Here's how the part is built. I have some questions about the finished solid (model axes, mm). Face numbers are marked on the shaded views. A direction names the side the tool comes from. Round coordinates to 2 decimals unless told otherwise and drop trailing zeros. Loops run counter-clockwise (first coordinate to the right, second up) from the corner with the lowest first, then second, coordinate; pieces in that order, holes last. Notation, with made-up numbers: M -28,64.25 L -9,64.25 A4 cw -9,68.25 Z; hole C 2.25,89 d10. An arc over 180 degrees is marked long. Answer as a JSON object with one key per item and string values.
Autodesk Fusion 360 part; units mm, degrees
sketch "Sketch1" plane through (0, 0, 0) normal (0, 0, 1) x (1, 0, 0)
  line L0 (0, 0) -> (110, 0)
  line L1 (110, 0) -> (110, 60)
  line L2 (110, 60) -> (0, 60)
  line L3 (0, 60) -> (0, 0)
  line L4 (0, 60) -> (110, 60)
  line L5 (110, 60) -> (110, 35)
  line L6 (110, 35) -> (0, 35)
  line L7 (0, 35) -> (0, 60)
  line L8 (75, 25) -> (35, 25)
  line L9 (35, 25) -> (35, 0)
  line L10 (75, 0) -> (75, 25)
  line L11 (75, 25) -> (35, -25) construction
  line L12 (35, 25) -> (75, -25) construction
  point P0 (55, 0)
  dimension "d12" = 110
  dimension "d13" = 60
  dimension "d14" = 110
  dimension "d15" = 25
  dimension "d16" = 40
  dimension "d17" = 50
extrude "Extrude1" add sketch "Sketch1" along normal blind 30 contours L0 L1 L3 L6 L8 L9 L10
extrude "Extrude2" add sketch "Sketch1" along normal blind 80 contours L1 L2 L3 L4 L5 L6 L7
fillet "Fillet1" radius 6 2 edges at (110, 47.5, 80) (0, 47.5, 80)
chamfer "Chamfer1" distance 3 angle 45 4 edges at (110, 0, 15) (75, 0, 15) (35, 0, 15) (0, 0, 15)
sketch "Sketch2" plane through (0, 35, 0) normal (0, -1, 0) x (1, 0, 0)
  arc A0 (6, 80) -> (0, 74) centre (6, 74) ccw
  line L0 (0, 74) -> (0, 30)
  line L1 (0, 30) -> (110, 30)
  line L2 (110, 30) -> (110, 74)
  arc A1 (110, 74) -> (104, 80) centre (104, 74) ccw
  line L3 (104, 80) -> (6, 80)
  line L4 (55, 80) -> (55, 30) construction
  circle A2 centre (80, 55) radius 6
  circle A3 centre (80, 55) radius 3
  circle A4 centre (30, 55) radius 6
  circle A5 centre (30, 55) radius 3
  dimension "d27" = 12
  dimension "d28" = 6
  dimension "d29" = 25
  dimension "d32" = 25
extrude "Extrude3" cut sketch "Sketch2" against normal blind 25 contours A3 | A5
extrude "Extrude4" cut sketch "Sketch2" against normal blind 5 contours A4
extrude "Extrude5" cut sketch "Sketch2" against normal blind 5 contours A2
equation "width = 60 mm"
equation "length = 110 mm"
equation "base_height = 30 mm"
equation "back_height = 80 mm"
equation "back_width = 25 mm"
equation "countersink_diameter = 12 mm"
equation "hole_diameter = 6 mm"
equation "countersink_depth = 5 mm"
equation "cut_depth = 25 mm"
equation "cut_width = 40 mm"
equation "d12 = length"
equation "d13 = width"
equation "d14 = length"
equation "d15 = back_width"
equation "d16 = cut_width"
equation "d17 = cut_depth * 2"
equation "top_radius = 6 mm"
equation "d19 = base_height"
equation "d21 = back_height"
equation "d24 = top_radius"
equation "chamfer = 3 mm"
equation "d26 = chamfer"
equation "d27 = countersink_diameter"
equation "d28 = hole_diameter"
equation "d29 = hole_distance_from_top"
equation "hole_distance_from_top = 25 mm"
equation "distance_between_holes = 50 mm"
equation "d32 = distance_between_holes / 2"
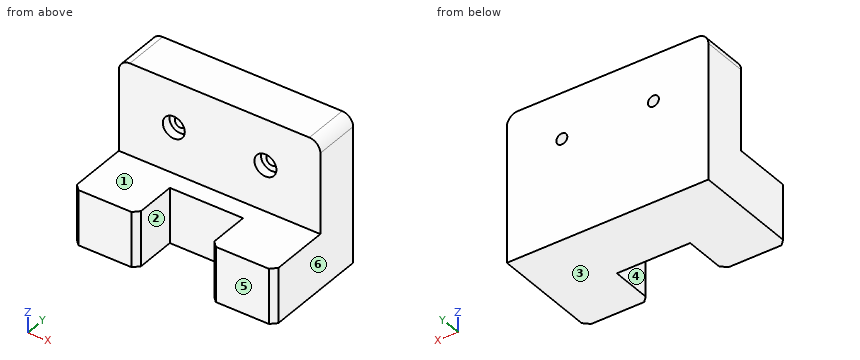
Item 1: I want a section at C-C, the plane y = 38.5. Please give me the cut outline in (x, z).
Resolved:
{"outline": "M 0,0 L 110,0 L 110,74 A6 ccw 104,80 L 6,80 A6 ccw 0,74 Z; hole C 30,55 d12; hole C 80,55 d12"}
Item 2: I want a section at A-A, the plane x = 30. Please give me the cut outline in (y, z), then the cut area to 3 significant figures.
Resolved:
{"outline": "M 0,0 L 60,0 L 60,52 L 40,52 L 40,49 L 35,49 L 35,30 L 0,30 Z; M 35,61 L 40,61 L 40,58 L 60,58 L 60,80 L 35,80 Z", "area": "2,870 mm²"}
Item 3: I'm going to push flat-ended pins straight in: pin 1 Ø3 at (x, z) = (56.5, 20) entering from -Y; pin 2 Ø3.5 at (x, z) = (31.5, 55.5) entering from -Y; pin 3 Ø4 at (x, z) = (20.5, 68) entering from -Y. Where does each tip first touch, or does it pass through?
Resolved:
{"pin 1": "y = 25", "pin 2": "y = 40", "pin 3": "y = 35"}
Item 4: On a 3-axis mill with a long thin cutter (end or side, diameter ignored), from which of +Z, -Z, +X, -X, +Y, -Y can I reach the whole of each face in a straight line? I mean the marked faces 1, 2 and 3. Say none if no direction works.
Resolved:
{"face 1": "+Z, +X, -X, -Y", "face 2": "+Z, -Z, -Y", "face 3": "-Z, +X, -X, +Y, -Y"}
Item 5: If we mould it in two halves opening along X, with no side actions, what happens to the marked faces 4, 5 and 6? For each: pulls with the +X half, pulls with the -X half, needs draft (parallel to the pull), parting line crosses it, or undercut.
Resolved:
{"face 4": "undercut", "face 5": "needs draft", "face 6": "pulls with the +X half"}
Item 6: I want a section at B-B, the plane z = 55. Please give me the cut outline in (x, y), then the cut area to 3 significant figures.
Resolved:
{"outline": "M 0,35 L 24,35 L 24,40 L 27,40 L 27,60 L 0,60 Z; M 33,40 L 36,40 L 36,35 L 74,35 L 74,40 L 77,40 L 77,60 L 33,60 Z; M 83,40 L 86,40 L 86,35 L 110,35 L 110,60 L 83,60 Z", "area": "2,390 mm²"}
Item 7: I want a section at D-D, the plane x = 72. Please give me the cut outline in (y, z), then the cut area to 3 significant figures.
Resolved:
{"outline": "M 25,0 L 60,0 L 60,80 L 35,80 L 35,30 L 25,30 Z", "area": "2,300 mm²"}
Item 8: Please list where these lines run through material, in increasing order: probe 1 along X at (y, z) = (6.5, 6.5); probe 2 along Z at (x, y) = (30, 51); probe 3 along Y at (x, z) = (67, 35.5). Write a range as from..to.
Resolved:
{"probe 1": "0..35, 75..110", "probe 2": "0..52, 58..80", "probe 3": "35..60"}
